Model file for the job. Use its own axes, mm. A direction names the side the tool comes from. Round coordinates to 2 decimals unless told otherwise and drop trailing zeros. Write each loop counter-clockwise with the first axis right and the second up, starting at its lowest first coordinate (ties: lowest second). Pieces come first, ordered by that corner, then holes. Notation, with made-up numbers: (39, 37) - (61, 37) arc R24 ccw to (61, 76) - close; hole circle Ø10 at (62, 34.5). An arc over 180 degrees is marked (long way). One line per item, written item: value.
from build123d import *

# Parameters (mm, degrees)
SKETCH1_R               = 5
CUT_EXTRUDE1_DEPTH      = 187.102122647
CUT_EXTRUDE1_DEPTH_BACK = 187.102122647
SKETCH2_W               = 140
SKETCH2_H               = 170
SKETCH4_R               = 2.5
CUT_EXTRUDE2_DEPTH      = 5


with BuildPart() as part:
    # Sketch1 → Revolve1 (revolve)
    with BuildSketch(Plane.XZ.offset(48)):
        with Locations((0, 20)):
            Circle(SKETCH1_R)
    revolve(axis=Axis((-43.255842548, -48, -55), (1, 0, 0)))

    # Sketch2 → Cut-Extrude1 (cut, two sides: drawn at the far end of the back side and taken through both)
    with BuildSketch(Plane(origin=(0, 0, 0), x_dir=(0, 0, -1), z_dir=(1, 0, 0)).offset(-CUT_EXTRUDE1_DEPTH_BACK)):
        with Locations((70, -50)):
            Rectangle(SKETCH2_W, SKETCH2_H)
    extrude(amount=CUT_EXTRUDE1_DEPTH + CUT_EXTRUDE1_DEPTH_BACK, mode=Mode.SUBTRACT)

    # Sketch4 → Cut-Extrude2 (cut)
    with BuildSketch(Plane.XY):
        Circle(SKETCH4_R)
        with Locations((0, -96)):
            Circle(SKETCH4_R)
    extrude(amount=CUT_EXTRUDE2_DEPTH, mode=Mode.SUBTRACT)


solid = part.part
1. Mould opens along Y. For faces 3 (the face through (0, 4, 0)), 4 (the face through (-0.54, -2.44, 2.46)) say: released by +Y, released by -Y, zero draft, split by the parting line, or undercut.
Report:
face 3: zero draft
face 4: undercut
2. Band-saw the part on A-A on x = 0. Write the cut outline in (y, z), plus the area to 3 significant figures.
Report:
outline: (-106.09, 0) - (-98.5, 0) - (-98.5, 5) - (-93.5, 5) - (-93.5, 0) - (-91.3, 0) arc R70 cw to (-4.7, 0) - (-2.5, 0) - (-2.5, 5) - (2.5, 5) - (2.5, 0) - (10.09, 0) arc R80 ccw to start
area: 1,070 mm²
3. Wall check: probe 1 along Y at (x, z) = (0, 3.55); probe 2 along Y at (x, z) = (0, 3.5); probe 3 along Y at (x, z) = (3.5, 8.5). Give the ranges that are in metal, low to high. Write a range as [from, to].
Report:
probe 1: [-102.52, -98.5], [-93.5, -86.37], [-9.63, -2.5], [2.5, 6.52]
probe 2: [-102.57, -98.5], [-93.5, -86.44], [-9.56, -2.5], [2.5, 6.57]
probe 3: [-94.27, -80.71], [-15.29, -1.73]
4. Drop flat-ended pins along their axis: pin 1 (4.5 mm diameter, centred on x = 0, y = -96, fed in from -Z); pin 2 (6 mm diameter, centred on y = -76, z = 18.5, fed in from -X); pin 3 (4 mm diameter, centred on x = -0.5, y = -87, fed in from +Z). Give the stop position or say it passes through.
Report:
pin 1: z = 5
pin 2: x = -4.96
pin 3: z = 15.91
5. Tool access for faces 1 (the face through (-0.33, -93.52, 2.46)), 2 (the face through (0, -99, 0)): list every direction of +Z, -Z, +X, -X, +Y, -Y with a clear straight run to the whole face (end or side of a thin tool).
Report:
face 1: -Z
face 2: -Z, +X, -X, +Y, -Y
